Could you check a few things on this model? Use its own coordinates, in mm. A direction names the side the tool comes from. Round coordinates to 2 decimals unless told otherwise and drop trailing zeros. Write each loop counter-clockwise with the first axis right and the second up, starting at its lowest first coordinate (ties: lowest second). Pieces come first, ordered by that corner, then holes. Notation, with made-up numbers: (39.5, -33) -> (49.5, -33) arc R26 cw to (49.5, -10) -> close; hole circle Ø7 at (41.25, -7). An arc over 180 degrees is marked (long way). Return JSON: item names as keys, results as strings.
Autodesk Inventor part; units mm, degrees
ref_plane "YZ Plane" through (0, 0, 0) normal (1, 0, 0) x (0, 1, 0)
ref_plane "XZ Plane" through (0, 0, 0) normal (0, 1, 0) x (-1, 0, 0)
ref_plane "XY Plane" through (0, 0, 0) normal (0, 0, 1) x (1, 0, 0)
sketch "Sketch_1" plane through (0, 0, 0) normal (0, 0, 1) x (1, 0, 0)
  line L0 (5, 0) -> (-7.8, 0)
  line L1 (-7.8, 0) -> (-7.8, 5)
  line L2 (-7.8, 5) -> (-5, 5)
  line L3 (-5, 5) -> (-5, 3)
  line L4 (-5, 3) -> (0, 3)
  line L5 (0, 3) -> (0, 2)
  line L6 (0, 2) -> (4.5705, 2)
  line L7 (4.5705, 2) -> (5, 1.5705)
  line L8 (5, 1.5705) -> (5, 0)
  line L9 (5, 0) -> (-7.8, 0)
revolve "Revolution1" add sketch "Sketch_1" angle 360 about axis through (5, 0, 0) along (1, 0, 0)
thread "Thread1"
sketch "Sketch_2" plane through (-7.8, 0, 0) normal (-1, 0, 0) x (0, 1, 0)
  line L0 (-1.4434, 0) -> (-0.7217, -1.25)
  line L1 (-0.7217, -1.25) -> (0.7217, -1.25)
  line L2 (0.7217, -1.25) -> (1.4434, 0)
  line L3 (1.4434, 0) -> (0.7217, 1.25)
  line L4 (0.7217, 1.25) -> (-0.7217, 1.25)
  line L5 (-0.7217, 1.25) -> (-1.4434, 0)
extrude "Extrusion1" cut sketch "Sketch_2" against normal blind 2.5
sketch "Sketch_3" plane through (0, 0, 0) normal (0, 0, 1) x (1, 0, 0)
  line L0 (-4.5783, 0) -> (-5.3, 0)
  line L1 (-5.3, 0) -> (-5.3, 1.25)
  line L2 (-5.3, 1.25) -> (-4.5783, 0)
  line L3 (-4.5783, 0) -> (-5.3, 0)
revolve "Revolution2" cut sketch "Sketch_3" angle 360 about axis through (-4.5783, 0, 0) along (1, 0, 0)
sketch "スケッチ4" plane through (5, 0, 0) normal (1, 0, 0) x (0, 0, -1)
  circle A0 centre (0, 0) radius 5
extrude "押し出し2" cut sketch "スケッチ4" against normal blind 2
properties part number "DBS4-5-5_AddProc"
1) Will these pins go through, and if not, where does the flat tip stop? pin 1 Ø3 at (x, y) = (-6.5, 3) entering from -Z; pin 2 Ø2 at (x, y) = (-5, 1.5) entering from +Z; pin 3 Ø3 at (x, z) = (0.5, 2) entering from +Y.
Return value:
{"pin 1": "z = -4.77", "pin 2": "z = 4.97", "pin 3": "y = 2.94"}
2) I want a section at D-D, the plane z = 1.5. Please give me the cut outline in (x, y), and give its area (3 significant figures).
Return value:
{"outline": "(-7.8, -4.77) -> (-5, -4.77) -> (-5, -2.6) -> (0, -2.6) -> (0, -1.32) -> (3, -1.32) -> (3, 1.32) -> (0, 1.32) -> (0, 2.6) -> (-5, 2.6) -> (-5, 4.77) -> (-7.8, 4.77) -> close", "area": "60.6 mm²"}
3) I want a section at A-A, the plane x = -5.5. Please give me the cut outline in (y, z).
Return value:
{"outline": "circle Ø10 at (0, 0); hole (-1.44, 0) -> (-0.72, -1.25) -> (0.72, -1.25) -> (1.44, 0) -> (0.72, 1.25) -> (-0.72, 1.25) -> close"}
4) I want a section at C-C, the plane x = -3.5. Please give me the cut outline in (y, z), and give its area (3 significant figures).
Return value:
{"outline": "circle Ø6 at (0, 0)", "area": "28.3 mm²"}
5) If I drill on probe 1 along X at (y, z) = (2.5, 2.5); probe 2 along Y at (x, z) = (-6.75, 0.5); probe 3 along X at (y, z) = (-1.75, 1.75), over which ranges is the centre line in solid material (lowest first)? Write a range as [from, to].
Return value:
{"probe 1": "[-7.8, -5]", "probe 2": "[-4.97, -1.15], [1.15, 4.97]", "probe 3": "[-7.8, 0]"}
6) For faces 1 (the face through (-6.568, -1.088, 0.616)), 2 (the face through (-7.8, 1.04, -1.04)), 3 (the face through (2, 0, -2)), which set-ups out of +Z, -Z, +X, -X, +Y, -Y let a thin tool reach every point of the face, with its end or its side?
Return value:
{"face 1": "-X", "face 2": "+Z, -Z, -X, +Y, -Y", "face 3": "+X"}
7) I want a section at B-B, the plane z = -2.25. Please give me the cut outline in (x, y).
Return value:
{"outline": "(-7.8, -4.47) -> (-5, -4.47) -> (-5, -1.98) -> (0, -1.98) -> (0, 1.98) -> (-5, 1.98) -> (-5, 4.47) -> (-7.8, 4.47) -> close"}
8) Thinking about a two-plate mould opening in Z: for faces 4 (the face through (-2, -3, 0)), 5 (the face through (0, 1, -2)), 6 (the face through (-7, 0, 1.25)), which applies, pulls with the +Z half, pulls with the -Z half, needs draft (parallel to the pull), parting line crosses it, or undercut?
Return value:
{"face 4": "parting line crosses it", "face 5": "needs draft", "face 6": "undercut"}
